from build123d import *

# Parameters (mm, degrees)
SKETCH1_R           = 5
BOSS_EXTRUDE1_DEPTH = 5
SKETCH2_R           = 2.25
BOSS_EXTRUDE2_DEPTH = 42.5
SKETCH3_R           = 1.25
CUT_EXTRUDE1_DEPTH  = 10
CHAMFER1_SIZE       = 2.5


with BuildPart() as part:
    # Sketch1 → Boss-Extrude1 (new body)
    with BuildSketch(Plane.XY):
        Circle(SKETCH1_R)
    extrude(amount=BOSS_EXTRUDE1_DEPTH)

    # Sketch2 → Boss-Extrude2 (add)
    with BuildSketch(Plane.XY.offset(5)):
        Circle(SKETCH2_R)
    extrude(amount=BOSS_EXTRUDE2_DEPTH)

    # Sketch3 → Cut-Extrude1 (cut)
    with BuildSketch(Plane.XY.offset(47.5)):
        Circle(SKETCH3_R)
    extrude(amount=-CUT_EXTRUDE1_DEPTH, mode=Mode.SUBTRACT)

    # Chamfer1
    chamfer1_edges = [part.edges().sort_by_distance(p)[0] for p in [
        (-5, 0, 0),
    ]]
    chamfer(chamfer1_edges, length=CHAMFER1_SIZE)


solid = part.part
Can you work these out from the model? Positions are in its coordinate system, mm. A direction names the side the tool comes from. Round coordinates to 2 decimals unless told otherwise and drop trailing zeros. Loops run counter-clockwise (first coordinate to the right, second up) from the corner with the lowest first, then second, coordinate; pieces in that order, holes last. Notation, with made-up numbers: (74.25, 85) - (101.25, 85) arc R34 cw to (101.25, 120) - close; hole circle Ø6 at (16.25, 46.5). An arc over 180 degrees is marked (long way). Use CSV: the item, a comma, the result in double quotes. Start each with the question number.
1) Please list where these lines run through material, in increasing order: probe 1 along Y at (x, z) = (0, 41.25); probe 2 along Z at (x, y) = (-3.75, 0.25); probe 3 along Z at (x, y) = (1.5, -1.75). Write a range as [from, to].
2) For faces 4 (the cylindrical face through (-0.29, 2.23, 25.95)), 5 (the flat face through (0, 0, 0)), which set-ups out of +Z, -Z, +X, -X, +Y, -Y let a thin tool reach every point of the face, with its end or its side?
3) If we section it at A-A on x = 0: Write out the boundary of the cut face in (y, z), plus the area to 3 significant figures.
4) If we section it at C-C on z = 42: Write out the boundary of the cut face in (x, y).
5) We'd pull the mould along X, two halves only. Please class faces 1 (the flat face through (2.2, -1, 5)), 2 (the cylindrical face through (-1.08, -4.88, 3.73)), 3 (the cylindrical face through (-0.27, -1.22, 42.57)): released by +X, released by -X, zero draft, split by the parting line, or undercut.
6) If we section it at D-D on z = 10.5: Write out the boundary of the cut face in (x, y), plus the area to 3 significant figures.
7) For pin 1 Ø2 at (x, y) = (-3.5, -1.5) entering from -Z; pin 2 Ø2 at (x, z) = (1.5, 8) entering from -Y; pin 3 Ø3 at (y, z) = (2.5, 8.5) entering from -X, each with a flat end and sliding along its axis, tell me the tip position at first contact or that it passes through.
Geometry results:
1,probe 1,"y = [-2.25, -1.25], [1.25, 2.25]"
1,probe 2,"z = [1.26, 5]"
1,probe 3,"z = [0, 5]"
2,face 4,"+Z"
2,face 5,"-Z, +X, -X, +Y, -Y"
3,outline,"(-5, 2.5) - (-2.5, 0) - (2.5, 0) - (5, 2.5) - (5, 5) - (2.25, 5) - (2.25, 47.5) - (1.25, 47.5) - (1.25, 37.5) - (-1.25, 37.5) - (-1.25, 47.5) - (-2.25, 47.5) - (-2.25, 5) - (-5, 5) - close"
3,area,"210 mm2"
4,outline,"circle Ø4.5 at (0, 0); hole circle Ø2.5 at (0, 0)"
5,face 1,"zero draft"
5,face 2,"split by the parting line"
5,face 3,"undercut"
6,outline,"circle Ø4.5 at (0, 0)"
6,area,"15.9 mm2"
7,pin 1,"stops at z = 0.31"
7,pin 2,"stops at y = -2.19"
7,pin 3,"stops at x = -2.02"
